Can you work these out from the model? Positions are in its coordinate system, mm. A direction names the side the tool comes from. Coordinates: 2 decimals unless noted, no trailing zeros. Order: outer loops, then holes, each group sorted by start corner. A loop starts at its lowest first (then second) coordinate and runs counter-clockwise, first axis right, second up.
```python
from build123d import *

# Parameters (mm, degrees)
EXTRUDE_1_DEPTH         = 60
CUT_EXTRUDE1_DEPTH      = 130.259429056
CUT_EXTRUDE1_DEPTH_BACK = 130.259429056
SKETCH1_R               = 2.1


with BuildPart() as part:
    # 草图1 → 凸台-拉伸1 (new body)
    with BuildSketch(Plane.XY):
        Polygon((0, 0), (0, 2), (102, 2), (102, -52), (0, -52), (0, -50), (100, -50), (100, 0), align=None)
    extrude(amount=EXTRUDE_1_DEPTH)

    # Sketch1 → Cut-Extrude1 (cut, two sides: drawn at the far end of the back side and taken through both)
    with BuildSketch(Plane(origin=(0, 0, 0), x_dir=(1, 0, 0), z_dir=(0, 1, 0)).offset(-CUT_EXTRUDE1_DEPTH_BACK)):
        with Locations(Location((6, -10, 0), (0, 0, 270))):
            Circle(SKETCH1_R)
        with Locations(Location((34, -10, 0), (0, 0, 270))):
            Circle(SKETCH1_R)
        with Locations(Location((34, -50, 0), (0, 0, 270))):
            Circle(SKETCH1_R)
        with Locations(Location((6, -50, 0), (0, 0, 270))):
            Circle(SKETCH1_R)
    extrude(amount=CUT_EXTRUDE1_DEPTH + CUT_EXTRUDE1_DEPTH_BACK, mode=Mode.SUBTRACT)


solid = part.part
```
1. Thinking about a two-plate mould opening in X: for faces 3 (the cylindrical face through (6.631, -51.014, 52.003)), 4 (the flat face through (66, -51, 60)), 5 (the flat face through (0, 1, 30)), which applies, pulls with the +X half, pulls with the -X half, needs draft (parallel to the pull), parting line crosses it, or undercut?
Completed:
face 3: undercut
face 4: needs draft
face 5: pulls with the -X half
2. Please list where these lines run through material, in increasing order: probe 1 along X at (y, z) = (-51.3, 50); probe 2 along Z at (x, y) = (6, 0.8); probe 3 along Y at (x, z) = (91, 9.5).
Completed:
probe 1: x = 0 to 3.9, 8.1 to 31.9, 36.1 to 102
probe 2: z = 0 to 7.9, 12.1 to 47.9, 52.1 to 60
probe 3: y = -52 to -50, 0 to 2
3. Imagine slicing it at B-B on x = 6. Please give me the cut outline in (y, z).
Completed:
outline: (-52, 0) - (-50, 0) - (-50, 7.9) - (-52, 7.9) - close; (-52, 12.1) - (-50, 12.1) - (-50, 47.9) - (-52, 47.9) - close; (-52, 52.1) - (-50, 52.1) - (-50, 60) - (-52, 60) - close; (0, 0) - (2, 0) - (2, 7.9) - (0, 7.9) - close; (0, 12.1) - (2, 12.1) - (2, 47.9) - (0, 47.9) - close; (0, 52.1) - (2, 52.1) - (2, 60) - (0, 60) - close
4. Imagine slicing it at A-A on z = 50. Please give me the cut outline in (x, y).
Completed:
outline: (0, -52) - (3.9, -52) - (3.9, -50) - (0, -50) - close; (0, 0) - (3.9, 0) - (3.9, 2) - (0, 2) - close; (8.1, -52) - (31.9, -52) - (31.9, -50) - (8.1, -50) - close; (8.1, 0) - (31.9, 0) - (31.9, 2) - (8.1, 2) - close; (36.1, -52) - (102, -52) - (102, 2) - (36.1, 2) - (36.1, 0) - (100, 0) - (100, -50) - (36.1, -50) - close
5. I'm going to push a flat-ended pin straight in: pin 1 (8 mm diameter, centred on y = -44, z = 38, fed in from -X). Where does the tip first touch, or does it pass through?
Completed:
pin 1: stops at x = 100
6. Imagine slicing it at C-C on x = 25. Please give me the cut outline in (y, z), then the cut area to 3 significant figures.
Completed:
outline: (-52, 0) - (-50, 0) - (-50, 60) - (-52, 60) - close; (0, 0) - (2, 0) - (2, 60) - (0, 60) - close
area: 240 mm2
7. On a 3-axis mill with a long thin cutter (end or side, diameter ignored), from which of +Z, -Z, +X, -X, +Y, -Y can I reach the whole of each face in a straight line? I mean faces 1 (the flat face through (51, 0, 30)), 2 (the flat face through (0, -51, 30)). Say none if no direction works.
Completed:
face 1: +Z, -Z, -X
face 2: +Z, -Z, -X, +Y, -Y
8. Imagine slicing it at D-D on z = 39.5. Please give me the cut outline in (x, y).
Completed:
outline: (0, -52) - (102, -52) - (102, 2) - (0, 2) - (0, 0) - (100, 0) - (100, -50) - (0, -50) - close
